from build123d import *

# Parameters (mm, degrees)
SKETCH_1_W             = 200
SKETCH_1_H             = 109
EXTRUDE_1_DEPTH        = 50
SKETCH_2_W             = 18.460680343
SKETCH_2_H             = 63.94452195
CUT_EXTRUDE_1_DEPTH    = 34
SKETCH_3_W             = 20.806626264
SKETCH_3_H             = 5.638388786
EXTRUDE_2_DEPTH        = 5
PATTERN_LINEAR_1_COUNT = 5
PATTERN_LINEAR_1_PITCH = 10


with BuildPart() as part:
    # 草图1 → 凸台-拉伸1 (new body)
    with BuildSketch(Plane(origin=(0, 0, 0), x_dir=(1, 0, 0), z_dir=(0, 1, 0))):
        with Locations((94.587973274, -49.622494432)):
            Rectangle(SKETCH_1_W, SKETCH_1_H)
    extrude(amount=EXTRUDE_1_DEPTH)

    # 草图2 → 切除-拉伸1 (cut)
    with BuildSketch(Plane(origin=(0, 50, 0), x_dir=(1, 0, 0), z_dir=(0, 1, 0))):
        with Locations((3.818313446, -46.706785098)):
            Rectangle(SKETCH_2_W, SKETCH_2_H)
    extrude(amount=-CUT_EXTRUDE_1_DEPTH, mode=Mode.SUBTRACT)

    # 草图3 → 凸台-拉伸2 (add)
    with BuildSketch(Plane(origin=(0, 16, 0), x_dir=(1, 0, 0), z_dir=(0, 1, 0))):
        with Locations((4.991286406, -25.341462736)):
            Rectangle(SKETCH_3_W, SKETCH_3_H)
    extrude_2 = extrude(amount=EXTRUDE_2_DEPTH)

    # 阵列(线性)1: 凸台-拉伸2 ×5
    with Locations(*[(0, 0, i * PATTERN_LINEAR_1_PITCH) for i in range(1, PATTERN_LINEAR_1_COUNT)]):
        add(extrude_2)


solid = part.part
Verification items for the finished model (mm, model axes). A direction names the side the tool comes from. Coordinates: 2 decimals unless noted, no trailing zeros. Order: outer loops, then holes, each group sorted by start corner. A loop starts at its lowest first (then second) coordinate and runs counter-clockwise, first axis right, second up. Notation, with made-up numbers: (72.25, 38.25) -> (119.25, 38.25) arc R17 ccw to (119.25, 51.25) -> close; hole circle Ø5 at (42, 67). An arc over 180 degrees is marked (long way). Use CSV: the item, a comma, the result in double quotes. Start each with the question number.
Q1. Depth check by flat-ended pin: P1, Ø3.5, axis at x = 1.5, z = 39.5, coming from the +Y side; P2, Ø10, axis at y = 35.5, z = 36, coming from the -X side; P3, Ø3.5, axis at x = 1.5, z = 50, coming from the +Y side. Enter the tip coordinate at first touch or a pass-through.
Q2. Section check A-A, the plane z = 60.5. Record the cut outline in (x, y).
Q3. Draft check along Z on faces 1 (the flat face through (194.588, 25, 50)), 2 (the flat face through (93, 25, 104.122)), 3 (the flat face through (4, 21, 55)). Enter one of: +Z half, -Z half, draft (parallel to the pull), parting line (faces both ways), or undercut.
Q4. Section check B-B, the plane y = 46. Record the cut outline in (x, z).
Q5. Tool access check on faces 4 (the flat face through (-5.412, 14, 50)), 5 (the flat face through (4, 18, 48.161)). Record the directions out of +Z, -Z, +X, -X, +Y, -Y that give a thin tool (end or side, any length) a straight path to the whole face; none if there is none.
Q6. Thickness scan on line 1 along X through (y, z) = (29.5, 54); line 2 along Y through (x, z) = (8, 63). Record the ranges inside material, lowest first.
Returned:
1,P1,"stops at y = 21"
1,P2,"stops at x = 13.05"
1,P3,"stops at y = 16"
2,outline,"(-5.41, 0) -> (194.59, 0) -> (194.59, 50) -> (13.05, 50) -> (13.05, 16) -> (-5.41, 16) -> close"
3,face 1,"draft"
3,face 2,"+Z half"
3,face 3,"undercut"
4,outline,"(-5.41, -4.88) -> (194.59, -4.88) -> (194.59, 104.12) -> (-5.41, 104.12) -> (-5.41, 78.68) -> (13.05, 78.68) -> (13.05, 14.73) -> (-5.41, 14.73) -> close"
5,face 4,"+Z, -Z, -X, +Y, -Y"
5,face 5,"-X, +Y"
6,line 1,"x = 13.05 to 194.59"
6,line 2,"y = 0 to 21"
